from build123d import *

# Parameters (mm, degrees)
F0_W      = 108.1741899252
F0_H      = 93.3166369796
F1_DEPTH  = 152.7411602437
F2_W      = 28.2202102244
F2_H      = 21.6964222491
F3_DEPTH  = 81.1772439629
F4_W      = 29.056660831
F4_H      = 19.965454936
F5_DEPTH  = 82.1499973536
F6_W      = 23.9808671176
F6_H      = 19.7158064693
F7_DEPTH  = 84.9992781878
F8_W      = 29.0753766894
F8_H      = 23.8046133891
F9_DEPTH  = 78.1470183283
F11_D     = 6.35
F13_D     = 6.35
F14_DEPTH = 28.7660323083
F16_D     = 6.35
F17_W     = 32.1477130055
F17_H     = 30.0406292081
F18_DEPTH = 95.8115551621


with BuildPart() as f1:
    # F0 (on Front) → F1 (new body)
    with BuildSketch(Plane.XZ):
        with Locations((9.279049933, 7.7308379114)):
            Rectangle(F0_W, F0_H)
    extrude(amount=F1_DEPTH)

    # F2 (on face) → F3 (join)
    with BuildSketch(Plane(origin=(-44.8080450296, 0, 0), x_dir=(0, -1, 0), z_dir=(-1, 0, 0))):
        with Locations((138.6310551316, 43.5409452766)):
            Rectangle(F2_W, F2_H)
    extrude(amount=F3_DEPTH)

    # F4 (on face) → F5 (join)
    with BuildSketch(Plane(origin=(-44.8080450296, 0, 0), x_dir=(0, -1, 0), z_dir=(-1, 0, 0))):
        with Locations((14.5283304155, 44.4064289331)):
            Rectangle(F4_W, F4_H)
    extrude(amount=F5_DEPTH)

    # F6 (on face) → F7 (join)
    with BuildSketch(Plane(origin=(-44.8080450296, 0, 0), x_dir=(0, -1, 0), z_dir=(-1, 0, 0))):
        with Locations((140.7507266849, -29.0695773438)):
            Rectangle(F6_W, F6_H)
    extrude(amount=F7_DEPTH)

    # F8 (on face) → F9 (join)
    with BuildSketch(Plane(origin=(-44.8080450296, 0, 0), x_dir=(0, -1, 0), z_dir=(-1, 0, 0))):
        with Locations((14.5376883447, -27.0251738839)):
            Rectangle(F8_W, F8_H)
    extrude(amount=F9_DEPTH)

    # F11 (through all)
    with Locations(Plane(origin=(0, 0, -38.9274805784), x_dir=(1, 0, 0), z_dir=(0, 0, -1))):
        with Locations((63.3661448956, 113.0213215947)):
            Hole(F11_D / 2)

    # F13 (through all)
    with Locations(Plane(origin=(0, 0, -38.9274805784), x_dir=(1, 0, 0), z_dir=(0, 0, -1))):
        with Locations((63.3661448956, 29.2834546417)):
            Hole(F13_D / 2)

    # F0 (on Front) + F9_face1 (on face) → F14 (join)
    with BuildSketch(Plane.XZ):
        with Locations((9.279049933, 7.7308379114)):
            Rectangle(F0_W, F0_H)
    with BuildSketch(Plane(origin=(-14.9495070386, 0, 7.3997359), x_dir=(-1, 0, 0), z_dir=(0, 1, 0))):
        Polygon((112.0085353446, 46.9894205011), (-78.3156519342, 46.9894205011), (-78.3156519342, -46.3272164785), (108.0055563193, -46.3272164785), (108.0055563193, -22.5226030894), (29.858537991, -22.5226030894), (29.858537991, 27.0239655651), (112.0085353446, 27.0239655651), align=None)
    extrude(amount=F14_DEPTH, dir=(0, -1, 0))

    # F16 (through all)
    with Locations(Plane(origin=(0, 0, -38.9274805784), x_dir=(1, 0, 0), z_dir=(0, 0, -1))):
        with Locations((0, 113.3106648922)):
            Hole(F16_D / 2)

    # F17 (on face) → F18 (cut)
    with BuildSketch(Plane.XY.offset(54.3891564012)):
        with Locations((16.0738565028, -72.7889351547)):
            Rectangle(F17_W, F17_H)
    extrude(amount=-F18_DEPTH, mode=Mode.SUBTRACT)


solid = f1.part
Part model, mm, in its own coordinate system. A direction names the side the tool comes from. Coordinates: 2 decimals unless noted, no trailing zeros. Write each loop counter-clockwise with the first axis right and the second up, starting at its lowest first coordinate (ties: lowest second). Pieces come first, ordered by that corner, then holes. Notation, with made-up numbers: M -36.5,-30 L -28.5,-30 A28 ccw -28.5,-7 Z; hole C -30,9 d6. An arc over 180 degrees is marked long. Return JSON: item names as keys, results as strings.
1. Probe L1, parallel to Y at x = 31.5, z = 41.5; L2, parallel to Z at x = -106.5, y = -133; L3, parallel to X at y = -61, z = 19.5. List the from-to ranges inside material, lowest first.
Determined:
{"L1": "-152.74 to -87.81, -57.77 to 0", "L2": "-38.93 to -19.21, 32.69 to 54.39", "L3": "-44.81 to 0, 32.15 to 63.37"}
2. Saw through at B-B, the plane x = 29. Write the cut outline in (y, z), then the cut area to 4 significant figures.
Determined:
{"outline": "M -152.74,-38.93 L -87.81,-38.93 L -87.81,54.39 L -152.74,54.39 Z; M -57.77,-38.93 L 0,-38.93 L 0,54.39 L -57.77,54.39 Z", "area": "11,450 mm²"}
3. Flat gauge pins, fed straight in: pin 1 Ø9 at (y, z) = (-76, 23.5) entering from -X; pin 2 Ø22 at (y, z) = (-19, 40.5) entering from -X; pin 3 Ø4 at (x, y) = (0, -113.31) entering from -Z. Where does each tip first touch, or does it go through?
Determined:
{"pin 1": "x = -44.81", "pin 2": "x = -126.96", "pin 3": "through"}
4. Saw through at C-C, the plane x = -98.5. Write the cut outline in (y, z), then the cut area to 3 significant figures.
Determined:
{"outline": "M -152.74,-38.93 L -128.76,-38.93 L -128.76,-19.21 L -152.74,-19.21 Z; M -152.74,32.69 L -124.52,32.69 L -124.52,54.39 L -152.74,54.39 Z; M -29.08,-38.93 L 0,-38.93 L 0,-15.12 L -29.08,-15.12 Z; M -29.06,34.42 L 0,34.42 L 0,54.39 L -29.06,54.39 Z", "area": "2,360 mm²"}
5. 3-axis set-ups, long thin cutter, end or side, ignore diameter. For faces 1 (the face through (-85, -29.057, 44)), 2 (the face through (-122.955, -14, -27)), 3 (the face through (-87, -141, -19.212)), 4 (the face through (16, -57.769, 8)): which of +Z, -Z, +X, -X, +Y, -Y reach the whole face in a straight line?
Determined:
{"face 1": "+Z, -Z, -X", "face 2": "-Z, -X, +Y", "face 3": "-X, -Y", "face 4": "+Z, -Z"}
6. Pull direction Z, two halves, no side cores. Call faces 5 (the face through (-10, -75, -38.927)), 6 (the face through (-44.808, -75, 7)), 7 (the face through (16, -87.809, 8)): pulls with the +Z half, pulls with the -Z half, needs draft (parallel to the pull), parting line crosses it, or undercut.
Determined:
{"face 5": "pulls with the -Z half", "face 6": "undercut", "face 7": "needs draft"}
7. Saw through at A-A, the plane y = -70.5. Write the cut outline in (x, z), then the cut area to 3 significant figures.
Determined:
{"outline": "M -44.81,-38.93 L 0,-38.93 L 0,54.39 L -44.81,54.39 Z; M 32.15,-38.93 L 63.37,-38.93 L 63.37,54.39 L 32.15,54.39 Z", "area": "7,090 mm²"}
8. Saw through at D-D, the plane z = 47. Write the cut outline in (x, y) (3 decimals).
Determined:
{"outline": "M -126.958,-29.057 L -44.808,-29.057 L -44.808,-124.521 L -125.985,-124.521 L -125.985,-152.741 L 63.366,-152.741 L 63.366,-116.196 A3.175 cw 63.366,-109.846 L 63.366,-32.458 A3.175 cw 60.234,-28.766 L 63.366,-28.766 L 63.366,0 L -126.958,0 Z; hole C 0,-113.311 d6.35; hole M 0,-87.809 L 32.148,-87.809 L 32.148,-57.769 L 0,-57.769 Z"}
